from build123d import *

# Parameters (mm, degrees)
F0_W      = 46
F0_H      = 12
F1_DEPTH  = 5
F2_W      = 8
F2_H      = 50
F3_DEPTH  = 1
F3_FACE_W = 8
F3_FACE_H = 50
F4_DEPTH  = 50
F5_W      = 12
F5_H      = 5
F6_DEPTH  = 12
F7_W      = 12
F7_H      = 5
F8_DEPTH  = 12
F11_W     = 40.896876
F11_H     = 40.029949
F12_DEPTH = 46.001
F13_W     = 8
F13_H     = 40.103398
F14_DEPTH = 25


with BuildPart() as f1:
    # F0 (on Top) → F1 (new body)
    with BuildSketch(Plane.XY):
        Rectangle(F0_W, F0_H)
    extrude(amount=F1_DEPTH)

    # F2 (on face) → F3 (join)
    with BuildSketch(Plane.XZ.offset(6)):
        with Locations((19, -20)):
            Rectangle(F2_W, F2_H)
    extrude(amount=F3_DEPTH)

    # F3_face (on face) → F4 (join)
    with BuildSketch(Plane(origin=(19, -7, -20), x_dir=(1, 0, 0), z_dir=(0, -1, 0))):
        Rectangle(F3_FACE_W, F3_FACE_H)
    extrude(amount=F4_DEPTH)

    # F5 (on face) → F6 (join)
    with BuildSketch(Plane.XZ.offset(6)):
        with Locations((-17, 2.5)):
            Rectangle(F5_W, F5_H)
    extrude(amount=F6_DEPTH)

    # F7 (on face) → F8 (join)
    with BuildSketch(Plane.XZ.offset(6)):
        with Locations((9, 2.5)):
            Rectangle(F7_W, F7_H)
    extrude(amount=F8_DEPTH)

    # F11 (on face) → F12 (cut, through all)
    with BuildSketch(Plane.YZ.offset(23)):
        with Locations((-26.551562, -25.014974)):
            Rectangle(F11_W, F11_H)
    extrude(amount=-F12_DEPTH, mode=Mode.SUBTRACT)

    # F13 (on face) → F14 (cut)
    with BuildSketch(Plane(origin=(0, -6, 0), x_dir=(-1, 0, 0), z_dir=(0, 1, 0))):
        with Locations((-19, -24.948301)):
            Rectangle(F13_W, F13_H)
    extrude(amount=-F14_DEPTH, mode=Mode.SUBTRACT)


solid = f1.part
Geometry: final body of the model. Coordinates: model frame, mm. A direction names the side the tool comes from. Give positions to 0.01 mm unless a question says otherwise; leave off trailing zeros. Write each loop counter-clockwise with the first axis right and the second up, starting at its lowest first coordinate (ties: lowest second). Pieces come first, ordered by that corner, then holes.
(1) Ray query, line 1 (X direction, y = -8, z = 1); line 2 (Z direction, x = 18, y = -2); line 3 (X direction, y = -50, z = -37). Return the intervals inside material, ascending.
(2) Access query for faces 5 (the flat face through (5, -11, 5)), 6 (the flat face through (-4, -6, 2)), 7 (the flat face through (19, -6, -2)), 8 (the flat face through (19, -52, -45)), 9 (the flat face through (-17, -18, 3)). Directions: +Z, -Z, +X, -X, +Y, -Y. A direction counts if a zero-diameter tool reaches every point of the face in a straight line with its end or side. Return the directions, or none.
(3) Cut plane B-B, the plane z = -4. Return loops of the section in (x, y), then the cut area to 3 significant figures.
(4) First-contact query: P1, Ø2, axis at x = 0, y = -5.5, coming from the -Z side; P2, Ø5.5, axis at x = 11, z = 1.5, coming from the -Y side; P3, Ø1.5, axis at x = 21, z = -1.5, coming from the +Y side. Flat tips, straight axial feed; report the tip coordinate or a pass-through.
(5) Cut plane C-C, the plane y = -34.5. Return loops of the section in (x, z).
(6) Mould query, pull axis X, two halves, no side actions, for faces 1 (the flat face through (-23, -6, 2)), 2 (the flat face through (-11, -12, 2)), 3 (the flat face through (3, -12, 2)), 4 (the flat face through (0, 6, 2)). Classes: released by +X, released by -X, zero draft, split by the parting line, or undercut.
(7) Cut plane A-A, the plane x = 18.5. Return loops of the section in (y, z).
Values follow:
1. line 1: x = -23 to -11, 3 to 23
1. line 2: z = 0 to 5
1. line 3: x = 15 to 23
2. face 5: +Z, +X, -X, +Y, -Y
2. face 6: +Z, -Z, -Y
2. face 7: -Z, +X, -X, +Y
2. face 8: -Z, +X, -X, +Y, -Y
2. face 9: +Z, -Z, -X, -Y
3. outline: (15, -57) - (23, -57) - (23, -6) - (15, -6) - close
3. area: 408 mm2
4. P1: stops at z = 0
4. P2: stops at y = -18
4. P3: stops at y = -6
5. outline: (15, -5) - (23, -5) - (23, 5) - (15, 5) - close
6. face 1: released by -X
6. face 2: undercut
6. face 3: undercut
6. face 4: zero draft
7. outline: (-57, -45) - (-47, -45) - (-47, -5) - (-31, -5) - (-31, -4.9) - (-6, -4.9) - (-6, 0) - (6, 0) - (6, 5) - (-57, 5) - close
